Source: CAD feature listing. Evaluate the final solid. Frame: model axes, mm. Face numbers are marked on the shaded views. A direction names the side the tool comes from. Give positions to 0.01 mm unless a question says otherwise; leave off trailing zeros. Order: outer loops, then holes, each group sorted by start corner. A loop starts at its lowest first (then second) coordinate and runs counter-clockwise, first axis right, second up. Notation, with made-up numbers: M 47.25,65.25 L 91.25,65.25 A30 cw 91.25,88.25 Z; hole C 33.25,33.25 d6. An arc over 180 degrees is marked long. Use CSV: the item, a comma, the result in double quotes. Start each with the question number.
Item 1: Section query D-D on z = -18. Return loops of the section in (x, y), and give its area (3 significant figures).
Item 2: Section query A-A on x = 0. Return loops of the section in (y, z), and give its area (3 significant figures).
Item 3: First-contact query: pin 1 (10 mm diameter, centred on x = 12.5, y = 36.5, fed in from -Z); pin 2 (2 mm diameter, centred on y = 55.5, z = -1.5, fed in from -X). Flat tips, straight axial feed; report the tip coordinate or a pass-through.
Item 4: Ray query, probe 1 along Y at (x, z) = (-7, 18); probe 2 along Y at (x, z) = (24.5, -23); probe 3 along Z at (x, y) = (-3, 44.5). Return the intervals inside material, ascending. Write a range as from..to.
Item 5: Access query for the marked faces 1 and 2. Directions: +Z, -Z, +X, -X, +Y, -Y. A direction counts if a zero-diameter tool reaches every point of the face in a straight line with its end or side. Return the directions, or none.
Item 6: Section query C-C on y = 53. Return loops of the section in (x, z), and give its area (3 significant figures).
Item 7: Section query B-B on z = 0. Return loops of the section in (x, y), and give its area (3 significant figures).
from build123d import *

# Parameters (mm, degrees)
ESQUISSE2_W        = 62
ESQUISSE2_H        = 62
BOSS_EXTRU_1_DEPTH = 27
ESQUISSE3_R        = 24
BOSS_EXTRU_2_DEPTH = 3
ESQUISSE4_R        = 3.5
BOSS_EXTRU_3_DEPTH = 40


with BuildPart() as part:
    # Esquisse2 → Boss.-Extru.1 (new body)
    with BuildSketch(Plane(origin=(0, 0, 0), x_dir=(1, 0, 0), z_dir=(0, 1, 0))):
        Rectangle(ESQUISSE2_W, ESQUISSE2_H)
    extrude(amount=BOSS_EXTRU_1_DEPTH)

    # Esquisse3 → Boss.-Extru.2 (add)
    with BuildSketch(Plane(origin=(0, 27, 0), x_dir=(1, 0, 0), z_dir=(0, 1, 0))):
        with Locations(Location((0, 0, 0), (0, 0, 270))):
            Circle(ESQUISSE3_R)
    extrude(amount=BOSS_EXTRU_2_DEPTH)

    # Esquisse4 → Boss.-Extru.3 (add)
    with BuildSketch(Plane(origin=(0, 30, 0), x_dir=(1, 0, 0), z_dir=(0, 1, 0))):
        with Locations(Location((0, 0, 0), (0, 0, 270))):
            Circle(ESQUISSE4_R)
    extrude(amount=BOSS_EXTRU_3_DEPTH)


solid = part.part
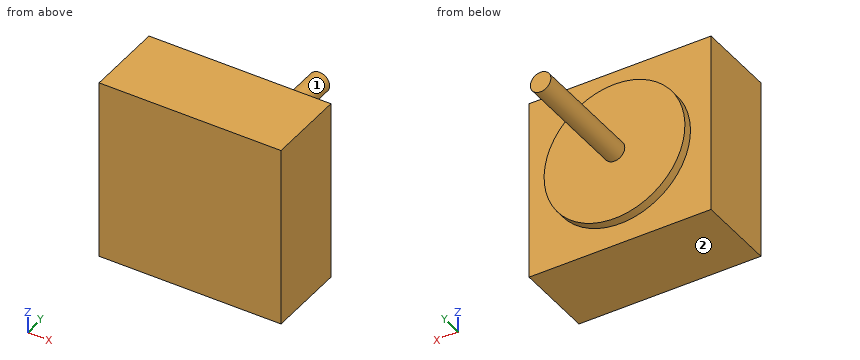
Verdict:
1,outline,"M -31,0 L 31,0 L 31,27 L 15.87,27 L 15.87,30 L -15.87,30 L -15.87,27 L -31,27 Z"
1,area,"1,770 mm2"
2,outline,"M 0,-31 L 27,-31 L 27,-24 L 30,-24 L 30,-3.5 L 70,-3.5 L 70,3.5 L 30,3.5 L 30,24 L 27,24 L 27,31 L 0,31 Z"
2,area,"2,100 mm2"
3,pin 1,"through"
3,pin 2,"x = -3.46"
4,probe 1,"0..30"
4,probe 2,"0..27"
4,probe 3,"-1.8..1.8"
5,face 1,"+Y"
5,face 2,"-Z, +X, -X, +Y, -Y"
6,outline,"C 0,0 d7"
6,area,"38.5 mm2"
7,outline,"M -31,0 L 31,0 L 31,27 L 24,27 L 24,30 L 3.5,30 L 3.5,70 L -3.5,70 L -3.5,30 L -24,30 L -24,27 L -31,27 Z"
7,area,"2,100 mm2"
